For this review, use the dimensioned drawing (mm, ordinates from the lowest corner) and the shaded views. A direction names the side the tool comes from. Coordinates: 2 decimals unless noted, no trailing zeros. Use CSV: the item, a comma, the result in double quotes.
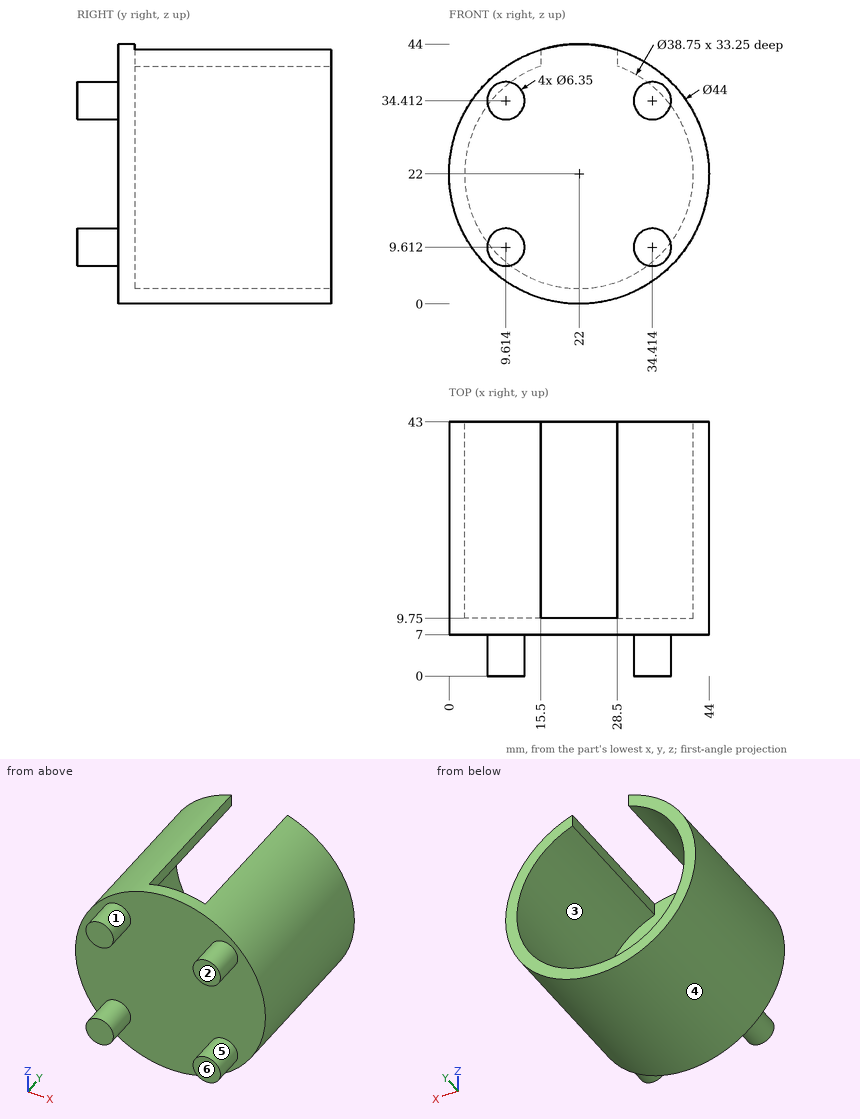
Item 1: For the marked faces 1, 2 and 3, list the 3-axis set-ups (+Z, -Z, +X, -X, +Y, -Y) from which the entire face can be reached by the end or side of a thin tool; tool diameter is ignored.
Solutions:
face 1,"-Y"
face 2,"+Z, -Z, +X, -X, -Y"
face 3,"+Y"
Item 2: To check wall thickness, follow line 1 along X through (y, z) = (24, 22) (1 decimal); line 2 along Z through (x, y) = (22, 28.5) (1 decimal); line 3 along Y through (x, z) = (17.5, 8). State the ranges of each line that lie inside material, in increasing order. Write a range as [from, to].
Solutions:
line 1,"[0, 2.6], [41.4, 44]"
line 2,"[0, 2.6]"
line 3,"[7, 9.75]"
Item 3: Clearance check with flat-ended pins moving along their axes: pin 1 Ø10 at (x, y) = (12, 4.5) entering from +Z; pin 2 Ø11.5 at (x, z) = (26.5, 14) entering from +Y; pin 3 Ø2 at (x, y) = (12, 4.5) entering from +Z. State where each tip first meets the part, or that it passes through.
Solutions:
pin 1,"z = 43.26"
pin 2,"y = 9.75"
pin 3,"z = 37.27"
Item 4: Draft analysis for pull direction X (two halves, no side actions). For the marked faces 4, 5 and 6, state which applies: released by +X, released by -X, zero draft, split by the parting line, or undercut.
Solutions:
face 4,"split by the parting line"
face 5,"undercut"
face 6,"zero draft"
